Build history of the part. All positions in model axes, mm. Round coordinates to 2 decimals unless told otherwise and drop trailing zeros. Write each loop counter-clockwise with the first axis right and the second up, starting at its lowest first coordinate (ties: lowest second). Pieces come first, ordered by that corner, then holes.
from build123d import *

# Parameters (mm, degrees)
F1_DEPTH = 18
F2_W     = 6
F2_H     = 366
F3_DEPTH = 6
F5_DEPTH = 10
F6_W     = 150
F6_H     = 20
F7_DEPTH = 20


with BuildPart() as f1:
    # F0 (on Right) → F1 (new body)
    with BuildSketch(Plane.YZ):
        Polygon((30, -907.5), (30, 722.5), (-30, 722.5), (-30, -497.5), (-430, -497.5), (-430, -907.5), align=None)
    extrude(amount=F1_DEPTH)

    # F2 (on face) → F3 (cut)
    with BuildSketch(Plane(origin=(0, 0, 0), x_dir=(0, -1, 0), z_dir=(-1, 0, 0))):
        with Locations((-9, -724.5)):
            Rectangle(F2_W, F2_H)
    extrude(amount=-F3_DEPTH, mode=Mode.SUBTRACT)

    # F4 (on face) → F5 (cut)
    with BuildSketch(Plane(origin=(0, 0, 0), x_dir=(0, -1, 0), z_dir=(-1, 0, 0))):
        with BuildLine():
            Line((394.488256, -576.120995), (388.705905, -577.670371))
            ThreePointArc((388.705905, -577.670371), (385.170371, -583.794095), (391.294095, -587.329629))
            Line((391.294095, -587.329629), (391.499671, -587.274545))
            Line((391.499671, -587.274545), (406.464466, -602.23934))
            ThreePointArc((406.464466, -602.23934), (417.200546, -604.472448), (423.529442, -595.517267))
            Line((423.529442, -595.517267), (425.090125, -550.825165))
            ThreePointArc((425.090125, -550.825165), (424.641241, -547.494139), (423.114034, -544.5))
            Line((423.114034, -544.5), (325, -544.5))
            ThreePointArc((325, -544.5), (320, -549.5), (325, -554.5))
            Line((325, -554.5), (414.955701, -554.5))
            Line((414.955701, -554.5), (413.535534, -595.168272))
            Line((413.535534, -595.168272), (394.488256, -576.120995))
        make_face()
    extrude(amount=-F5_DEPTH, mode=Mode.SUBTRACT)

    # F6 (on face) → F7 (join)
    with BuildSketch(Plane(origin=(0, 0, 0), x_dir=(0, -1, 0), z_dir=(-1, 0, 0))):
        with Locations((300, -529.5)):
            Rectangle(F6_W, F6_H)
    extrude(amount=F7_DEPTH)


solid = f1.part
1) Slice it at A-A (z = -619). Write the cut outline in (x, y).
Results:
outline: (0, -430) - (18, -430) - (18, 30) - (0, 30) - (0, 12) - (6, 12) - (6, 6) - (0, 6) - close
2) Wall check: L1, parallel to Z at x = 4.5, y = -364.5; L2, parallel to X at y = -77.5, z = -557; L3, parallel to Z at x = -13, y = -352. Give the ranges that are in metal, low to high.
Results:
L1: z = -907.5 to -554.5, -544.5 to -497.5
L2: x = 0 to 18
L3: z = -539.5 to -519.5
3) Slice it at B-B (y = -255.5). Write the cut outline in (x, z), plus the area to 3 significant figures.
Results:
outline: (-20, -539.5) - (0, -539.5) - (0, -907.5) - (18, -907.5) - (18, -497.5) - (0, -497.5) - (0, -519.5) - (-20, -519.5) - close
area: 7,780 mm2
4) Slice it at C-C (x = -11). Write the cut outline in (y, z), plus the area to 3 significant figures.
Results:
outline: (-375, -539.5) - (-225, -539.5) - (-225, -519.5) - (-375, -519.5) - close
area: 3,000 mm2
5) Slice it at D-D (y = -342). Write the cut outline in (x, z), plus the area to 3 significant figures.
Results:
outline: (-20, -539.5) - (0, -539.5) - (0, -544.5) - (10, -544.5) - (10, -554.5) - (0, -554.5) - (0, -907.5) - (18, -907.5) - (18, -497.5) - (0, -497.5) - (0, -519.5) - (-20, -519.5) - close
area: 7,680 mm2
6) Pin check, flat tips, straight feed: pin 1 Ø3 at (x, y) = (3.5, -378.5) entering from +Z; pin 2 Ø10 at (x, z) = (-11.5, -533.5) entering from -Y; pin 3 Ø6 at (x, y) = (-6, -271) entering from -Z. Stop position of each tip, or through.
Results:
pin 1: stops at z = -497.5
pin 2: stops at y = -375
pin 3: stops at z = -539.5
7) Mould opens along Y. For faces 1 (the flat face through (10, -384, -554)), 2 (the flat face through (0, -133, -511)) say: released by +Y, released by -Y, zero draft, split by the parting line, or undercut.
Results:
face 1: undercut
face 2: zero draft
